```python
from build123d import *

# Parameters (mm, degrees)
F0_R     = 23
F0_R_2   = 21
F1_DEPTH = 4.5
F2_DEPTH = 3
F3_R     = 0.99999


# Not quite as in the source:
# - a fillet or chamfer is up to 0.001 mm smaller than in the source, because OpenCascade refuses the exact size


with BuildPart() as f1:
    # F0 (on Top) → F1 (new body)
    with BuildSketch(Plane.XY):
        Circle(F0_R)
        Circle(F0_R_2, mode=Mode.SUBTRACT)
        Circle(F0_R_2)
    extrude(amount=-F1_DEPTH)

    # F0 (on Top) → F2 (cut)
    with BuildSketch(Plane.XY):
        Circle(F0_R_2)
    extrude(amount=-F2_DEPTH, mode=Mode.SUBTRACT)

    # F3 (radius 1 in the source; OpenCascade refuses exactly that, so slightly less here)
    f3_edges = [f1.edges().sort_by_distance(p)[0] for p in [
        (-21, 0, 0),
        (-23, 0, 0),
    ]]
    fillet(f3_edges, radius=F3_R)


solid = f1.part
```
Could you check a few things on this model? Use its own coordinates, in mm. Coordinates: 2 decimals unless noted, no trailing zeros. Write each loop counter-clockwise with the first axis right and the second up, starting at its lowest first coordinate (ties: lowest second). Pieces come first, ordered by that corner, then holes. Notation, with made-up numbers: M 75.5,37.25 L 128.5,37.25 A18 cw 128.5,53.25 Z; hole C 62.25,1 d8. An arc over 180 degrees is marked long. Answer as CSV lines item,"result". Start each with the question number.
1) For P1, Ø1, axis at y = 5, z = -1, coming from the +X side; P2, Ø1.5, axis at x = 2.5, z = -3.5, coming from the +Y side; P3, Ø1.5, axis at y = 13, z = -2.5, coming from the -X side, each with a flat end and sliding along its axis, tell me the tip position at first contact or that it passes through.
2) Please list where these lines run through material, in increasing order: line 1 (Y direction, x = 0, z = -1.7); line 2 (Z direction, x = -10, y = 1); line 3 (Y direction, x = 11, z = -2.6). Write a range as from..to.
3) I want a section at C-C, the plane z = -2.35. Please give me the cut outline in (x, y).
4) We'd pull the mould along Y, two halves only. Please class faces 1 (the flat face through (0, 0, -3)), 2 (the flat face through (0, 0, -4.5)), 3 (the cylindrical face through (-2.994, 22.804, -2.725)): +Y half, -Y half, draft (parallel to the pull), parting line (faces both ways), or undercut.
Data:
1,P1,"stops at x = 22.56"
1,P2,"stops at y = 22.93"
1,P3,"stops at x = -19.47"
2,line 1,"y = -23..-21, 21..23"
2,line 2,"z = -4.5..-3"
2,line 3,"y = -20.2..-17.89, 17.89..20.2"
3,outline,"C 0,0 d46; hole C 0,0 d42"
4,face 1,"undercut"
4,face 2,"draft"
4,face 3,"parting line"
